from build123d import *

# Parameters (mm, degrees)
SKETCH1_W           = 80
SKETCH1_H           = 53
BOSS_EXTRUDE1_DEPTH = 30
SKETCH2_W           = 76
SKETCH2_H           = 49
CUT_EXTRUDE1_DEPTH  = 28
CUT_EXTRUDE2_DEPTH  = 6
SKETCH4_W           = 37
SKETCH4_H           = 10
CUT_EXTRUDE3_DEPTH  = 6
SKETCH5_W           = 2.5
SKETCH5_H           = 2.5
STANDOFFS_DEPTH     = 4
FILLET3_R           = 5
FILLET4_R           = 5
SKETCH6_W           = 3
SKETCH6_H           = 45
BOTTOM_GRILL_DEPTH  = 2
CUT_EXTRUDE5_REACH  = 74.863
SKETCH7_W           = 2
SKETCH7_H           = 15
CUT_EXTRUDE6_START  = -53
SKETCH8_R           = 1.75
CUT_EXTRUDE6_DEPTH  = 53
SKETCH9_R           = 1.75
CUT_EXTRUDE7_DEPTH  = 2
SKETCH10_W          = 3
SKETCH10_H          = 20
SKETCH10_W_2        = 2
CUT_EXTRUDE8_DEPTH  = 2


with BuildPart() as part:
    # Sketch1 → Boss-Extrude1 (new body)
    with BuildSketch(Plane(origin=(0, 0, 0), x_dir=(1, 0, 0), z_dir=(0, 1, 0))):
        Rectangle(SKETCH1_W, SKETCH1_H)
    extrude(amount=BOSS_EXTRUDE1_DEPTH)

    # Sketch2 → Cut-Extrude1 (cut)
    with BuildSketch(Plane(origin=(0, 30, 0), x_dir=(1, 0, 0), z_dir=(0, 1, 0))):
        Rectangle(SKETCH2_W, SKETCH2_H)
    extrude(amount=-CUT_EXTRUDE1_DEPTH, mode=Mode.SUBTRACT)

    # Sketch3 → Cut-Extrude2 (cut)
    with BuildSketch(Plane(origin=(40, 0, 0), x_dir=(0, 0, -1), z_dir=(1, 0, 0))):
        with BuildLine():
            Line((6, 15), (6, 5))
            Line((6, 5), (-9, 5))
            Line((-9, 5), (-9, 15))
            ThreePointArc((-9, 15), (-1.5, 22.5), (6, 15))
        make_face()
    extrude(amount=-CUT_EXTRUDE2_DEPTH, mode=Mode.SUBTRACT)

    # Sketch4 → Cut-Extrude3 (cut)
    with BuildSketch(Plane.ZY.offset(40)):
        with Locations((0, 18)):
            Rectangle(SKETCH4_W, SKETCH4_H)
    extrude(amount=-CUT_EXTRUDE3_DEPTH, mode=Mode.SUBTRACT)

    # Sketch5 → Standoffs (add)
    with BuildSketch(Plane(origin=(0, 2, 0), x_dir=(1, 0, 0), z_dir=(0, 1, 0))):
        with Locations((36.75, 23.25)):
            Rectangle(SKETCH5_W, SKETCH5_H)
        with Locations((36.75, -23.25)):
            Rectangle(SKETCH5_W, SKETCH5_H)
        with Locations((-36.75, -23.25)):
            Rectangle(SKETCH5_W, SKETCH5_H)
        with Locations((-36.75, 23.25)):
            Rectangle(SKETCH5_W, SKETCH5_H)
    extrude(amount=STANDOFFS_DEPTH)

    # Fillet3
    fillet3_edges = [part.edges().sort_by_distance(p)[0] for p in [
        (-39, 23, -18.5),
    ]]
    fillet(fillet3_edges, radius=FILLET3_R)

    # Fillet4
    fillet4_edges = [part.edges().sort_by_distance(p)[0] for p in [
        (-39, 23, 18.5),
    ]]
    fillet(fillet4_edges, radius=FILLET4_R)

    # Sketch6 → Bottom Grill (cut)
    with BuildSketch(Plane.XZ):
        with Locations((33.5, 0)):
            Rectangle(SKETCH6_W, SKETCH6_H)
        with Locations((24.5, 0)):
            Rectangle(SKETCH6_W, SKETCH6_H)
        with Locations((15.5, 0)):
            Rectangle(SKETCH6_W, SKETCH6_H)
        with Locations((6.5, 0)):
            Rectangle(SKETCH6_W, SKETCH6_H)
        with Locations((-2.5, 0)):
            Rectangle(SKETCH6_W, SKETCH6_H)
        with Locations((-11.5, 0)):
            Rectangle(SKETCH6_W, SKETCH6_H)
    extrude(amount=-BOTTOM_GRILL_DEPTH, mode=Mode.SUBTRACT)

    # Cut-Extrude5: up to this face of the body (flat: up to its plane)
    cut_extrude5_end = Plane(part.part.faces().sort_by_distance((0, 15, 26.5))[0])
    # Sketch7 → Cut-Extrude5 (cut, up to the picked face)
    with BuildSketch(Plane(origin=(0, 0, -26.5), x_dir=(-1, 0, 0), z_dir=(0, 0, -1)), mode=Mode.PRIVATE) as cut_extrude5_sk1:
        with Locations((-33, 15)):
            Rectangle(SKETCH7_W, SKETCH7_H)
    cut_extrude5_tool1 = split(extrude(cut_extrude5_sk1.sketch, amount=-CUT_EXTRUDE5_REACH, mode=Mode.PRIVATE), bisect_by=cut_extrude5_end, keep=Keep.BOTH, mode=Mode.PRIVATE)
    # Sketch7 → Cut-Extrude5 (cut, up to the picked face)
    with BuildSketch(Plane(origin=(0, 0, -26.5), x_dir=(-1, 0, 0), z_dir=(0, 0, -1)), mode=Mode.PRIVATE) as cut_extrude5_sk2:
        with Locations((-25, 15)):
            Rectangle(SKETCH7_W, SKETCH7_H)
    cut_extrude5_tool2 = split(extrude(cut_extrude5_sk2.sketch, amount=-CUT_EXTRUDE5_REACH, mode=Mode.PRIVATE), bisect_by=cut_extrude5_end, keep=Keep.BOTH, mode=Mode.PRIVATE)
    # Sketch7 → Cut-Extrude5 (cut, up to the picked face)
    with BuildSketch(Plane(origin=(0, 0, -26.5), x_dir=(-1, 0, 0), z_dir=(0, 0, -1)), mode=Mode.PRIVATE) as cut_extrude5_sk3:
        with Locations((-17, 15)):
            Rectangle(SKETCH7_W, SKETCH7_H)
    cut_extrude5_tool3 = split(extrude(cut_extrude5_sk3.sketch, amount=-CUT_EXTRUDE5_REACH, mode=Mode.PRIVATE), bisect_by=cut_extrude5_end, keep=Keep.BOTH, mode=Mode.PRIVATE)
    # Sketch7 → Cut-Extrude5 (cut, up to the picked face)
    with BuildSketch(Plane(origin=(0, 0, -26.5), x_dir=(-1, 0, 0), z_dir=(0, 0, -1)), mode=Mode.PRIVATE) as cut_extrude5_sk4:
        with Locations((-9, 15)):
            Rectangle(SKETCH7_W, SKETCH7_H)
    cut_extrude5_tool4 = split(extrude(cut_extrude5_sk4.sketch, amount=-CUT_EXTRUDE5_REACH, mode=Mode.PRIVATE), bisect_by=cut_extrude5_end, keep=Keep.BOTH, mode=Mode.PRIVATE)
    # Sketch7 → Cut-Extrude5 (cut, up to the picked face)
    with BuildSketch(Plane(origin=(0, 0, -26.5), x_dir=(-1, 0, 0), z_dir=(0, 0, -1)), mode=Mode.PRIVATE) as cut_extrude5_sk5:
        with Locations((-1, 15)):
            Rectangle(SKETCH7_W, SKETCH7_H)
    cut_extrude5_tool5 = split(extrude(cut_extrude5_sk5.sketch, amount=-CUT_EXTRUDE5_REACH, mode=Mode.PRIVATE), bisect_by=cut_extrude5_end, keep=Keep.BOTH, mode=Mode.PRIVATE)
    # Sketch7 → Cut-Extrude5 (cut, up to the picked face)
    with BuildSketch(Plane(origin=(0, 0, -26.5), x_dir=(-1, 0, 0), z_dir=(0, 0, -1)), mode=Mode.PRIVATE) as cut_extrude5_sk6:
        with Locations((7, 15)):
            Rectangle(SKETCH7_W, SKETCH7_H)
    cut_extrude5_tool6 = split(extrude(cut_extrude5_sk6.sketch, amount=-CUT_EXTRUDE5_REACH, mode=Mode.PRIVATE), bisect_by=cut_extrude5_end, keep=Keep.BOTH, mode=Mode.PRIVATE)
    add(cut_extrude5_tool1.solids().sort_by(Axis((33, 15, -26.5), (0, 0, 1)))[0], mode=Mode.SUBTRACT)
    add(cut_extrude5_tool2.solids().sort_by(Axis((25, 15, -26.5), (0, 0, 1)))[0], mode=Mode.SUBTRACT)
    add(cut_extrude5_tool3.solids().sort_by(Axis((17, 15, -26.5), (0, 0, 1)))[0], mode=Mode.SUBTRACT)
    add(cut_extrude5_tool4.solids().sort_by(Axis((9, 15, -26.5), (0, 0, 1)))[0], mode=Mode.SUBTRACT)
    add(cut_extrude5_tool5.solids().sort_by(Axis((1, 15, -26.5), (0, 0, 1)))[0], mode=Mode.SUBTRACT)
    add(cut_extrude5_tool6.solids().sort_by(Axis((-7, 15, -26.5), (0, 0, 1)))[0], mode=Mode.SUBTRACT)

    # Sketch8 → Cut-Extrude6 (cut)
    with BuildSketch(Plane(origin=(0, 0, -26.5), x_dir=(-1, 0, 0), z_dir=(0, 0, -1)).offset(CUT_EXTRUDE6_START)):
        with Locations((-5, 26)):
            Circle(SKETCH8_R)
        with Locations((25, 26)):
            Circle(SKETCH8_R)
    extrude(amount=CUT_EXTRUDE6_DEPTH, mode=Mode.SUBTRACT)

    # Sketch9 → Cut-Extrude7 (cut)
    with BuildSketch(Plane.ZY.offset(40)):
        with Locations((-20.5, 26)):
            Circle(SKETCH9_R)
        with Locations((20.5, 26)):
            Circle(SKETCH9_R)
    extrude(amount=-CUT_EXTRUDE7_DEPTH, mode=Mode.SUBTRACT)

    # Sketch10 → Cut-Extrude8 (cut)
    with BuildSketch(Plane(origin=(40, 0, 0), x_dir=(0, 0, -1), z_dir=(1, 0, 0))):
        with Locations((20, 15)):
            Rectangle(SKETCH10_W, SKETCH10_H)
        with Locations((15, 15)):
            Rectangle(SKETCH10_W, SKETCH10_H)
        with Locations((10, 15)):
            Rectangle(SKETCH10_W, SKETCH10_H)
        with Locations((-21.5, 15)):
            Rectangle(SKETCH10_W_2, SKETCH10_H)
        with Locations((-17.5, 15)):
            Rectangle(SKETCH10_W_2, SKETCH10_H)
        with Locations((-13.5, 15)):
            Rectangle(SKETCH10_W_2, SKETCH10_H)
    extrude(amount=-CUT_EXTRUDE8_DEPTH, mode=Mode.SUBTRACT)


solid = part.part
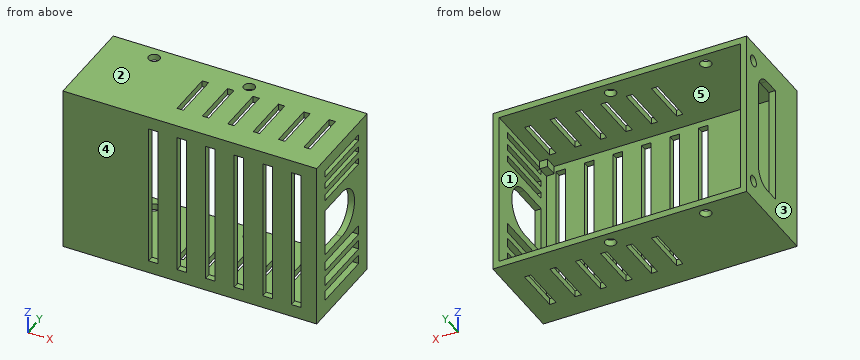
Work out the finished part from the listing and answer in its coordinate system (mm). Face numbers are marked on the shaded views. A direction names the side the tool comes from. Give positions to 0.01 mm unless a question says otherwise; leave off trailing zeros. Loops run counter-clockwise (first coordinate to the right, second up) from the corner with the lowest first, then second, coordinate; pieces in that order, holes last. Notation, with made-up numbers: M -15.75,86 L 11.25,86 A15 ccw 11.25,109 Z; hole C 87,15.5 d1. An arc over 180 degrees is marked long. Use CSV: the item, a comma, the result in double quotes.
1) Find section C-C on y = 26. Give the number of separate pieces and of enclosed holes in the cut face, plus the area to 3 significant figures.
Answer:
separate pieces,"6"
enclosed holes,"0"
area,"474 mm^2"
2) Find section D-D on x = -33. Write down the section's boundary in (y, z).
Answer:
outline,"M 0,-26.5 L 30,-26.5 L 30,-24.5 L 2,-24.5 L 2,24.5 L 30,24.5 L 30,26.5 L 0,26.5 Z"
3) Which of the six approach directions +Z, -Z, +X, -X, +Y, -Y give full straight-line access (tool end or side, diameter ignored) to the marked faces 4 and 5?
Answer:
face 4,"+Z, -Z, +X, -X, -Y"
face 5,"+Y"
4) Given P1, Ø2, axis at x = -36.5, z = 23, coming from the +Y side, flat-ended and moving along its own axis, determine where the tip first touches the part or whether it passes through.
Answer:
P1,"y = 6"
5) Find section B-B on x = -25. Write down the section's boundary in (y, z), plus the area to 3 significant figures.
Answer:
outline,"M 0,-26.5 L 24.25,-26.5 L 24.25,-24.5 L 2,-24.5 L 2,24.5 L 24.25,24.5 L 24.25,26.5 L 0,26.5 Z; M 27.75,-26.5 L 30,-26.5 L 30,-24.5 L 27.75,-24.5 Z; M 27.75,24.5 L 30,24.5 L 30,26.5 L 27.75,26.5 Z"
area,"204 mm^2"
6) Determine the mould class of the marked faces 1, 2 and 3 for opening direction Z: released by +Z, released by -Z, zero draft, split by the parting line, or undercut.
Answer:
face 1,"undercut"
face 2,"released by +Z"
face 3,"zero draft"
7) Find section A-A on y = 3.25. Write down the section's boundary in (x, z), plus the area to 3 significant figures.
Answer:
outline,"M -40,-26.5 L 40,-26.5 L 40,26.5 L -40,26.5 Z; hole M -38,-22 L -35.5,-22 L -35.5,-24.5 L 35.5,-24.5 L 35.5,-22 L 38,-22 L 38,22 L 35.5,22 L 35.5,24.5 L -35.5,24.5 L -35.5,22 L -38,22 Z"
area,"541 mm^2"
8) Consider L1, parallel to X at y = 26, z = -25.55; L2, parallel to X at y = 26.25, z = 11.5; L3, parallel to Y at x = -38.6, z = -20.5. Determine where each line is inside the solid, lowest interval first.
Answer:
L1,"-40 to -26.75, -23.25 to 3.25, 6.75 to 40"
L2,"-40 to -38, 38 to 40"
L3,"0 to 24.25, 27.75 to 30"
